from build123d import *

# Parameters (mm, degrees)
CROQUIS1_W              = 54
CROQUIS1_H              = 13
SALIENTE_EXTRUIR1_DEPTH = 10
CORTAR_EXTRUIR1_DEPTH   = 8
CROQUIS1_4_R            = 2.875
CORTAR_EXTRUIR2_DEPTH   = 11
CROQUIS2_W              = 50.887178886
CROQUIS2_H              = 27.662521268
CORTAR_EXTRUIR3_DEPTH   = 33.22


with BuildPart() as part:
    # Croquis1 → Saliente-Extruir1 (new body)
    with BuildSketch(Plane(origin=(0, 0, 0), x_dir=(1, 0, 0), z_dir=(0, 1, 0))):
        Rectangle(CROQUIS1_W, CROQUIS1_H)
    extrude(amount=SALIENTE_EXTRUIR1_DEPTH)

    # Croquis1<3> → Cortar-Extruir1 (cut)
    with BuildSketch(Plane(origin=(0, 0, 0), x_dir=(1, 0, 0), z_dir=(0, 1, 0))):
        Polygon((-18.33826859, -4.05), (-13.66173141, -4.05), (-11.32346282, 0), (-13.66173141, 4.05), (-18.33826859, 4.05), (-20.67653718, 0), align=None)
        Polygon((20.67653718, 0), (18.33826859, 4.05), (13.66173141, 4.05), (11.32346282, 0), (13.66173141, -4.05), (18.33826859, -4.05), align=None)
    extrude(amount=CORTAR_EXTRUIR1_DEPTH, mode=Mode.SUBTRACT)

    # Croquis1<4> → Cortar-Extruir2 (cut, through all)
    with BuildSketch(Plane(origin=(0, 0, 0), x_dir=(1, 0, 0), z_dir=(0, 1, 0))):
        with Locations((-16, 0)):
            Circle(CROQUIS1_4_R)
        with Locations((16, 0)):
            Circle(CROQUIS1_4_R)
    extrude(amount=CORTAR_EXTRUIR2_DEPTH, mode=Mode.SUBTRACT)

    # Croquis2 → Cortar-Extruir3 (cut, through all)
    with BuildSketch(Plane.ZY.offset(5.22)):
        with Locations((0.866942471, 5.460502056)):
            Rectangle(CROQUIS2_W, CROQUIS2_H)
    extrude(amount=-CORTAR_EXTRUIR3_DEPTH, mode=Mode.SUBTRACT)


solid = part.part
Work out the finished part from the listing and answer in its coordinate system (mm). A direction names the side the tool comes from. Give positions to 0.01 mm unless a question says otherwise; leave off trailing zeros. Write each loop counter-clockwise with the first axis right and the second up, starting at its lowest first coordinate (ties: lowest second). Pieces come first, ordered by that corner, then holes.
Q1. The part is cut by section C-C on z = -1.75. Give the vertices of the cut face in (x, y).
Answer:
outline: (-27, 0) - (-19.67, 0) - (-19.67, 8) - (-18.28, 8) - (-18.28, 10) - (-27, 10) - close; (-13.72, 8) - (-12.33, 8) - (-12.33, 0) - (-5.22, 0) - (-5.22, 10) - (-13.72, 10) - close
Q2. The part is cut by section B-B on y = 6.25. Give the vertices of the cut face in (x, z).
Answer:
outline: (-27, -6.5) - (-5.22, -6.5) - (-5.22, 6.5) - (-27, 6.5) - close; hole (-20.68, 0) - (-18.34, -4.05) - (-13.66, -4.05) - (-11.32, 0) - (-13.66, 4.05) - (-18.34, 4.05) - close
Q3. The part is cut by section A-A on x = -16. Give the vertices of the cut face in (y, z) (3 decimals), and give its area (3 significant figures).
Answer:
outline: (0, -6.5) - (10, -6.5) - (10, -2.875) - (8, -2.875) - (8, -4.05) - (0, -4.05) - close; (0, 4.05) - (8, 4.05) - (8, 2.875) - (10, 2.875) - (10, 6.5) - (0, 6.5) - close
area: 53.7 mm2
Q4. A tool of negligible diameter and unlimited length cuts with its end or side. For faces 5 (the face through (-19.491, 3.944, -2.053)), 6 (the face through (-13.258, 8.986, -0.864)), from which of +Z, -Z, +X, -X, +Y, -Y can it reach the whole face along a straight path? Write none if from no direction.
Answer:
face 5: -Y
face 6: +Y, -Y
Q5. For a pull along X with two mould halves and no side action, classify faces 1 (the face through (-12.48, 3.94, -2)), 2 (the face through (-27, 5, 0)), 3 (the face through (-16.3, 0, -4.4)), 4 (the face through (-12.509, 3.944, 2.053)) as released by +X, released by -X, zero draft, split by the parting line, or undercut.
Answer:
face 1: undercut
face 2: released by -X
face 3: zero draft
face 4: undercut
Q6. Straight lines are drawn through the part: L1, parallel to Z at x = -16, y = 8.9 (3 decimals); L2, parallel to Z at x = -14.5, y = 6; L3, parallel to Y at x = -20.25, z = 0.25. For each, find the intervals that lie inside material, in ascending order.
Answer:
L1: z = -6.5 to -2.875, 2.875 to 6.5
L2: z = -6.5 to -4.05, 4.05 to 6.5
L3: y = 8 to 10
